Work out the finished part from the listing and answer in its coordinate system (mm). Round coordinates to 2 decimals unless told otherwise and drop trailing zeros. Order: outer loops, then holes, each group sorted by start corner. A loop starts at its lowest first (then second) coordinate and runs counter-clockwise, first axis right, second up. Notation, with made-up numbers: (2.25, 42) - (8.25, 42) arc R36 ccw to (8.25, 78) - close; hole circle Ø6 at (-1.75, 20.25). An arc over 180 degrees is marked (long way). Use one line per item in the form item = value. Start each with the question number.
Q1. The part is cut by section C-C on z = 102.5. Determine the outline of the cut face in (x, y).
Q2. Find the intervals of material crossed by line 1 (Z direction, x = 2.8, y = 21.5); line 2 (Y direction, x = 0.95, z = 15); line 3 (Z direction, x = 1.9, y = 29.5), in increasing order. Write a range as [from, to].
Q3. The part is cut by section A-A on x = 1.95. Determine the outline of the cut face in (y, z).
Q4. The part is cut by section B-B on y = 25. Determine the outline of the cut face in (x, z).
Autodesk Inventor part; units mm, degrees
ref_plane "YZ Plane" through (0, 0, 0) normal (1, 0, 0) x (0, 1, 0)
ref_plane "XZ Plane" through (0, 0, 0) normal (0, 1, 0) x (-1, 0, 0)
ref_plane "XY Plane" through (0, 0, 0) normal (0, 0, 1) x (1, 0, 0)
sketch "スケッチ1" plane through (0, 0, 0) normal (1, 0, 0) x (0, 1, 0)
  line L0 (105, -75.231) -> (-35, 225)
  line L1 (-35, 225) -> (-105, 225)
  line L2 (-105, 225) -> (-105, -225)
  line L3 (-105, -225) -> (105, -225)
  line L4 (105, -225) -> (105, -75.231)
  line L5 (-147, 0) -> (147, 0)
  line L6 (0, -315) -> (0, 315)
  point P0 (0, 0)
  point P1 (-105, 0)
  point P2 (0, -225)
  dimension "d0" = 70
  dimension "d1" = 450
  dimension "d2" = 210
  dimension "d3" = 25
extrude "押し出し1" add sketch "スケッチ1" along normal blind 3
properties part number "side" material "CFRP"
Found:
q1.outline = (0, -105) - (3, -105) - (3, 22.12) - (0, 22.12) - close
q2.line_1 = [-225, 103.84]
q2.line_2 = [-105, 62.92]
q2.line_3 = [-225, 86.68]
q3.outline = (-105, -225) - (105, -225) - (105, -75.23) - (-35, 225) - (-105, 225) - close
q4.outline = (0, -225) - (3, -225) - (3, 96.33) - (0, 96.33) - close
